The figure shows three views and two pictorial views of one solid part (mm, origin at its lowest corner). Answer the questions. Coordinates: 2 decimals unless noted, no trailing zeros. Loops run counter-clockwise (first coordinate to the right, second up) from the corner with the lowest first, then second, coordinate; pieces in that order, holes last. Notation, with made-up numbers: (63, 55) -> (74, 55) arc R26 cw to (74, 86) -> close; hole circle Ø3 at (49.25, 4). An arc over 180 degrees is marked (long way). Answer as a JSON object with one key per item and string values. Group by question number.
1) Section C-C, the plane x = 61 is taken. Give the vertices of the cut face in (y, z), plus the area to 3 significant figures.
2) Flat-ended cylindrical pins translate along their axes: P1, Ø1, axis at y = 55.5, z = 2.5, coming from the +X side; P2, Ø1, axis at x = 30.5, z = 15, coming from the +Y side; P3, Ø8, axis at y = 71, z = 12.5, coming from the +X side. Find the tip coordinate at first contact, or state that the pin passes through.
3) Section B-B, the plane y = 50 is taken. Give the vertices of the cut face in (x, z), plus the area to 4 significant figures.
4) Section A-A, the plane z = 17.75 is taken. Give the vertices of the cut face in (x, y), plus the area to 3 significant figures.
5) Section D-D, the plane y = 13.5 is taken. Give the vertices of the cut face in (x, z), plus the area to 3 significant figures.
6) Determine the mould class of the marked faces 1 and 2 for opening direction X: released by +X, released by -X, zero draft, split by the parting line, or undercut.
7) Consider probe 1 along Y at (x, z) = (46, 11.75); probe 2 along Y at (x, z) = (20.5, 4.25); probe 3 along X at (y, z) = (75, 19.25) (1 decimal). Determine where each line is inside the solid, lowest interval first. Write a range as [from, to].
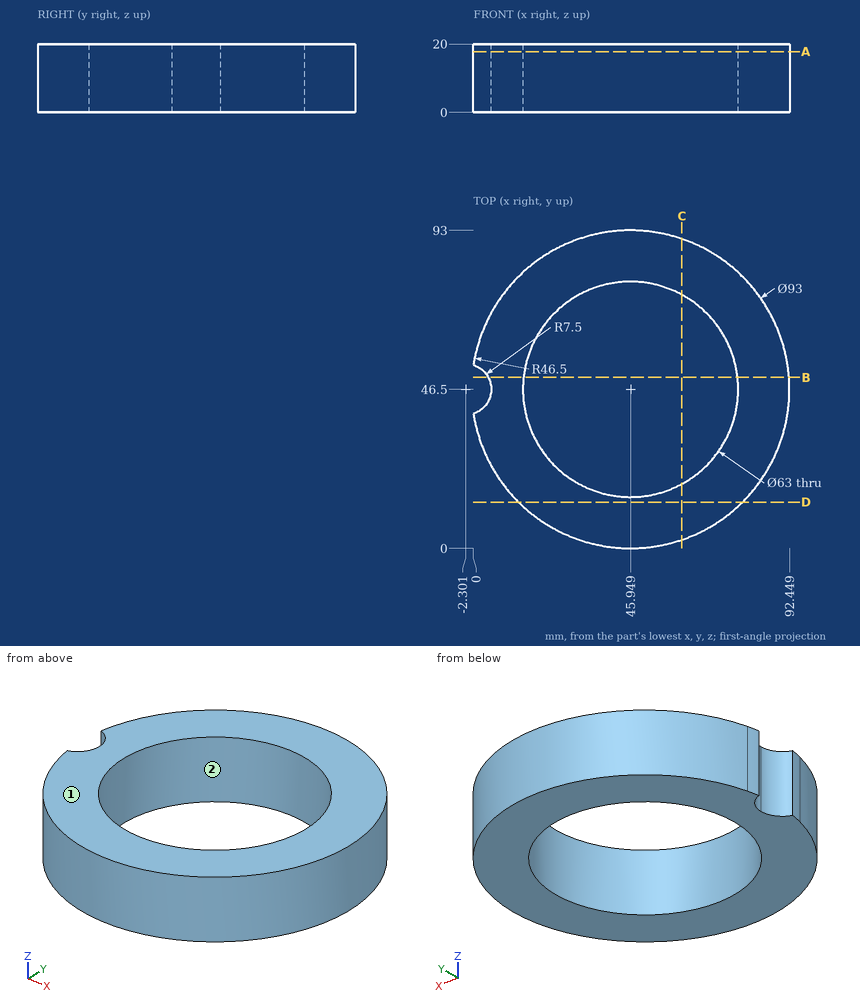
Determined:
{
 "1": {"outline": "(2.5, 0) -> (18.83, 0) -> (18.83, 20) -> (2.5, 20) -> close; (74.17, 0) -> (90.5, 0) -> (90.5, 20) -> (74.17, 20) -> close", "area": "653 mm²"},
 "2": {"P1": "x = 91.67", "P2": "y = 90.53", "P3": "x = 87.69"},
 "3": {"outline": "(4.33, 0) -> (14.64, 0) -> (14.64, 20) -> (4.33, 20) -> close; (77.25, 0) -> (92.32, 0) -> (92.32, 20) -> (77.25, 20) -> close", "area": "507.5 mm²"},
 "4": {"outline": "(0, 39.36) arc R46.5 ccw (long way) to (0, 53.64) arc R7.5 cw to start; hole circle Ø63 at (45.95, 46.5)", "area": "3,620 mm²"},
 "5": {"outline": "(13.19, 0) -> (78.71, 0) -> (78.71, 20) -> (13.19, 20) -> close", "area": "1,310 mm²"},
 "6": {"face 1": "zero draft", "face 2": "undercut"},
 "7": {"probe 1": "[0, 15], [78, 93]", "probe 2": "[7.58, 27.94], [65.06, 85.42]", "probe 3": "[9.2, 32.5], [59.4, 82.7]"}
}
